Geometry check sheet. Reference: the model listing, model coordinates, mm. Give positions to 0.01 mm unless a question says otherwise; leave off trailing zeros. Write each loop counter-clockwise with the first axis right and the second up, starting at its lowest first coordinate (ties: lowest second). Pieces come first, ordered by that corner, then holes. Notation, with made-up numbers: M 19.5,34 L 37.5,34 A20 cw 37.5,65 Z; hole C -30.75,1.25 d7. An arc over 180 degrees is marked long. Use one line per item in the form item = value. Start each with the question number.
```python
from build123d import *

# Parameters (mm, degrees)
SKETCH1_W           = 39.497
SKETCH1_H           = 71.501
SKETCH1_W_2         = 34.417
SKETCH1_H_2         = 66.421
SKETCH1_W_3         = 5.08
SKETCH1_H_3         = 10.16
BOSS_EXTRUDE1_DEPTH = 3.175
FILLET1_R           = 1.27


with BuildPart() as part:
    # Sketch1 → Boss-Extrude1 (new, symmetric)
    # profile 1 of 2: a face of its own
    with BuildSketch(Plane(origin=(0, 0, 0), x_dir=(0, 0, -1), z_dir=(1, 0, 0))):
        Rectangle(SKETCH1_W, SKETCH1_H)
        Rectangle(SKETCH1_W_2, SKETCH1_H_2, mode=Mode.SUBTRACT)
    # profile 2 of 2: a face of its own
    with BuildSketch(Plane(origin=(0, 0, 0), x_dir=(0, 0, -1), z_dir=(1, 0, 0))):
        with Locations((-22.2885, 30.6705)):
            Rectangle(SKETCH1_W_3, SKETCH1_H_3)
    extrude(amount=BOSS_EXTRUDE1_DEPTH, both=True)

    # Fillet1
    fillet1_edges = [part.edges().sort_by_distance(p)[0] for p in [
        (-3.175, -5.08, 19.7485),
        (-3.175, 25.5905, 22.2885),
        (-3.175, 30.6705, 24.8285),
        (-3.175, 35.7505, 2.54),
        (3.175, 33.2105, 0),
        (-3.175, 0, -19.7485),
        (-3.175, -35.7505, 0),
        (-3.175, 0, -17.2085),
        (-3.175, 33.2105, 0),
        (-3.175, 0, 17.2085),
        (-3.175, -33.2105, 0),
        (3.175, 0, -17.2085),
        (0, -35.7505, 19.7485),
        (0, 25.5905, 19.7485),
        (0, 25.5905, 24.8285),
        (0, -35.7505, -19.7485),
        (0, -33.2105, -17.2085),
        (0, 33.2105, -17.2085),
        (0, 33.2105, 17.2085),
        (0, -33.2105, 17.2085),
        (3.175, -35.7505, 0),
        (3.175, 0, -19.7485),
        (3.175, 35.7505, 2.54),
        (3.175, 30.6705, 24.8285),
        (3.175, 25.5905, 22.2885),
        (3.175, -5.08, 19.7485),
        (3.175, -33.2105, 0),
        (3.175, 0, 17.2085),
    ]]
    fillet(fillet1_edges, radius=FILLET1_R - 0.0001)  # a hair under: the kernel refuses the full size


solid = part.part
```
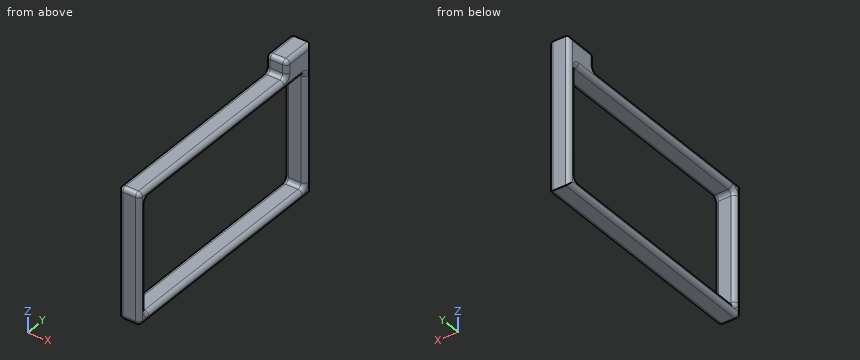
(1) Thickness scan on probe 1 along Z at (x, y) = (1, -6); probe 2 along Z at (x, y) = (1.25, 27.5); probe 3 along Y at (x, z) = (0, -4). Record the ranges inside material, lowest first. Write a range as [from, to].
(2) Depth check by flat-ended pin: pin 1 (1.1 mm diameter, centred on x = 0, y = 0, fed in from +Z); pin 2 (3 mm diameter, centred on x = 1, z = 22.5, fed in from -Y). Enter the tip coordinate at first touch or a pass-through.
(3) Sectioned sample at C-C, the plane x = -0.75. Record the boundary of the cut face in (y, z), plus the area to 3 significant figures.
Numbers:
q1.probe_1 = [-19.75, -17.21], [17.21, 19.75]
q1.probe_2 = [-19.75, -17.21], [17.21, 24.83]
q1.probe_3 = [-35.75, -33.21], [33.21, 35.75]
q2.pin_1 = 19.75
q2.pin_2 = 25.59
q3.outline = M -35.75,-18.48 A1.27 ccw -34.48,-19.75 L 35.75,-19.75 L 35.75,24.83 L 26.86,24.83 A1.27 ccw 25.59,23.56 L 25.59,21.02 A1.27 cw 24.32,19.75 L -34.48,19.75 A1.27 ccw -35.75,18.48 Z; hole M -33.21,-15.94 A1.27 ccw -31.94,-17.21 L 31.94,-17.21 A1.27 ccw 33.21,-15.94 L 33.21,15.94 A1.27 ccw 31.94,17.21 L -31.94,17.21 A1.27 ccw -33.21,15.94 Z
q3.area = 590 mm2
